from build123d import *

# Parameters (mm, degrees)
BOSS_EXTRUDE1_DEPTH = 10
CUT_EXTRUDE19_DEPTH = 10


with BuildPart() as part:
    # Sketch1 → Boss-Extrude1 (new body)
    with BuildSketch(Plane.XY):
        with BuildLine():
            Line((-50, 60), (50, 60))
            ThreePointArc((50, 60), (57.071067812, 57.071067812), (60, 50))
            Line((60, 50), (60, -50))
            ThreePointArc((60, -50), (57.071067812, -57.071067812), (50, -60))
            Line((50, -60), (-50, -60))
            ThreePointArc((-50, -60), (-57.071067812, -57.071067812), (-60, -50))
            Line((-60, -50), (-60, 50))
            ThreePointArc((-60, 50), (-57.071067812, 57.071067812), (-50, 60))
        make_face()
    extrude(amount=BOSS_EXTRUDE1_DEPTH)

    # Sketch2 → Cut-Extrude19 (cut)
    with BuildSketch(Plane.XY.offset(10)):
        Polygon((-29.461538462, 50), (19.256410256, 50), (19.256410256, 32.051282051), (-11.512820513, 32.051282051), (-11.512820513, 12.820512821), (19.256410256, 12.820512821), (19.256410256, -5.128205128), (-11.512820513, -5.128205128), (-11.512820513, -50), (-29.461538462, -50), align=None)
    extrude(amount=-CUT_EXTRUDE19_DEPTH, mode=Mode.SUBTRACT)


solid = part.part
Geometry check sheet. Reference: the model listing, model coordinates, mm. A direction names the side the tool comes from. Round coordinates to 2 decimals unless told otherwise and drop trailing zeros. Loops run counter-clockwise (first coordinate to the right, second up) from the corner with the lowest first, then second, coordinate; pieces in that order, holes last.
Item 1: Cross-section at A-A on x = -13. Record the boundary of the cut face in (y, z), then the cut area to 3 significant figures.
Item 2: Thickness scan on line 1 (Y direction, x = 18.5, z = 3); line 2 (Y direction, x = -12.5, z = 0.5); line 3 (X direction, y = -35, z = 6). Record the ranges inside material, lowest first.
Item 3: Cross-section at B-B on y = -31.5. Record the boundary of the cut face in (x, z).
Item 4: Access from +Z, -Z, +X, -X, +Y, -Y to the whole of each face (thin tool, end or side, straight path). Record for faces 1 (the flat face through (4, 12.821, 5)), 2 (the cylindrical face through (57.15, -56.99, 4.93)).
Item 5: Gauge pin test, flat ends, axial feed: pin 1 (10 mm diameter, centred on x = -20, y = 31.5, fed in from -Z); pin 2 (1 mm diameter, centred on x = -33, y = -7.5, fed in from -Z). Record the tip position at first contact, or that the pin passes through.
Item 6: Cross-section at D-D on x = 8.5. Record the boundary of the cut face in (y, z), then the cut area to 3 significant figures.
Item 7: Cross-section at C-C on z = 8.5. Record the boundary of the cut face in (x, y).
Answer sheet:
1. outline: (-60, 0) - (-50, 0) - (-50, 10) - (-60, 10) - close; (50, 0) - (60, 0) - (60, 10) - (50, 10) - close
1. area: 200 mm2
2. line 1: y = -60 to -5.13, 12.82 to 32.05, 50 to 60
2. line 2: y = -60 to -50, 50 to 60
2. line 3: x = -60 to -29.46, -11.51 to 60
3. outline: (-60, 0) - (-29.46, 0) - (-29.46, 10) - (-60, 10) - close; (-11.51, 0) - (60, 0) - (60, 10) - (-11.51, 10) - close
4. face 1: +Z, -Z
4. face 2: +Z, -Z, +X, -Y
5. pin 1: passes through
5. pin 2: stops at z = 0
6. outline: (-60, 0) - (-5.13, 0) - (-5.13, 10) - (-60, 10) - close; (12.82, 0) - (32.05, 0) - (32.05, 10) - (12.82, 10) - close; (50, 0) - (60, 0) - (60, 10) - (50, 10) - close
6. area: 841 mm2
7. outline: (-60, -50) arc R10 ccw to (-50, -60) - (50, -60) arc R10 ccw to (60, -50) - (60, 50) arc R10 ccw to (50, 60) - (-50, 60) arc R10 ccw to (-60, 50) - close; hole (-29.46, -50) - (-11.51, -50) - (-11.51, -5.13) - (19.26, -5.13) - (19.26, 12.82) - (-11.51, 12.82) - (-11.51, 32.05) - (19.26, 32.05) - (19.26, 50) - (-29.46, 50) - close
